Can you work these out from the model? Positions are in its coordinate system, mm. A direction names the side the tool comes from. Coordinates: 2 decimals unless noted, no trailing zeros. Loops run counter-clockwise (first coordinate to the right, second up) from the corner with the lowest first, then second, coordinate; pieces in that order, holes last. Notation, with made-up numbers: (59, 11) -> (86, 11) arc R32 cw to (86, 38) -> close; hole circle Ø7 at (-32, 2). An arc over 180 degrees is marked (long way). Use one line per item in the form item = value. Start each with the question number.
(1) I'm going to push flat-ended pins straight in: pin 1 (2 mm diameter, centred on y = -2, z = -18.5, fed in from +X); pin 2 (3 mm diameter, centred on y = 0, z = -3, fed in from +X); pin 3 (8 mm diameter, centred on y = -4.5, z = -2, fed in from -X); pin 4 (11.5 mm diameter, centred on x = 7, y = -1.5, fed in from -Z). Where does each tip first touch, or does it pass through?
(2) Imagine slicing it at C-C (x = -4). List the corners of the cut face in (y, z) for me.
(3) Imagine slicing it at A-A (z = -9). State how many separate pieces and enclosed holes the cut face has, plus the area to 3 significant figures.
(4) On a 3-axis mill with a long thin cutter (end or side, diameter ignored), from which of +Z, -Z, +X, -X, +Y, -Y can I reach the whole of each face in a straight line? I mean faces 1 (the flat face through (0, -9.5, -7)), 2 (the cylindrical face through (13.215, 9.199, -6.902)), 3 (the flat face through (5.5, -5, -22)), 4 (the flat face through (-6, -2, -7)). Say none if no direction works.
(5) Thinking about a two-plate mould opening in X: for faces 5 (the cylindrical face through (-14.45, -11.38, 1.52)), 6 (the flat face through (1.5, 5, -22)), 7 (the flat face through (1, 2, -6)), which applies, released by +X, released by -X, zero draft, split by the parting line, or undercut?
(6) I need wall thicknesses on line 1 (X direction, y = -7.5, z = -6); line 2 (Z direction, x = 18.5, y = 3.5); line 3 (X direction, y = 0.5, z = -15). Which ranges of each line are inside material? Lowest first, please. Write a range as [from, to].
(7) Imagine slicing it at B-B (z = -20). List the corners of the cut face in (x, y) for me.
(8) Imagine slicing it at D-D (x = 20). List the corners of the cut face in (y, z) for me, plus the area to 3 significant figures.
```python
from build123d import *
from OCP.BRepFilletAPI import BRepFilletAPI_MakeChamfer

# Parameters (mm, degrees)
SKIZZE1_R                       = 1.5
AUFSATZ_LINEAR_AUSTRAGEN1_DEPTH = 3
VERRUNDUNG1_R                   = 2
FASE1_SIZE                      = 1.5
AUFSATZ_LINEAR_AUSTRAGEN2_DEPTH = 2
AUFSATZ_LINEAR_AUSTRAGEN3_DEPTH = 14
SCHNITT_LINEAR_AUSTRAGEN1_DEPTH = 17
SKIZZE5_W                       = 24
SKIZZE5_H                       = 11
AUFSATZ_LINEAR_AUSTRAGEN4_DEPTH = 4
SKIZZE6_W                       = 3
SKIZZE6_H                       = 1
AUFSATZ_LINEAR_AUSTRAGEN5_DEPTH = 8
SKIZZE7_W                       = 2
SKIZZE7_H                       = 4
AUFSATZ_LINEAR_AUSTRAGEN6_DEPTH = 13
SKIZZE8_W                       = 2
SKIZZE8_H                       = 4
AUFSATZ_LINEAR_AUSTRAGEN7_DEPTH = 15
FASE2_SIZE                      = 2
FASE2_SIZE2                     = 0.75
VERRUNDUNG2_R                   = 0.25


with BuildPart() as part:
    # Skizze1 → Aufsatz-Linear austragen1 (new body)
    with BuildSketch(Plane.XY):
        with BuildLine():
            ThreePointArc((23.364069952, 3.949125596), (25.187731645, 0), (23.364069952, -3.949125596))
            Line((23.364069952, -3.949125596), (14.5, -11.5))
            Line((14.5, -11.5), (-14.5, -11.5))
            Line((-14.5, -11.5), (-23.364069952, -3.949125596))
            ThreePointArc((-23.364069952, -3.949125596), (-25.187731645, 0), (-23.364069952, 3.949125596))
            Line((-23.364069952, 3.949125596), (-14.5, 11.5))
            Line((-14.5, 11.5), (14.5, 11.5))
            Line((14.5, 11.5), (23.364069952, 3.949125596))
        make_face()
        with Locations((20, 0)):
            Circle(SKIZZE1_R, mode=Mode.SUBTRACT)
        with Locations((-20, 0)):
            Circle(SKIZZE1_R, mode=Mode.SUBTRACT)
    extrude(amount=AUFSATZ_LINEAR_AUSTRAGEN1_DEPTH)

    # Verrundung1
    verrundung1_edges = [part.edges().sort_by_distance(p)[0] for p in [
        (14.5, -11.5, 1.5),
        (-14.5, -11.5, 1.5),
        (-14.5, 11.5, 1.5),
        (14.5, 11.5, 1.5),
    ]]
    fillet(verrundung1_edges, radius=VERRUNDUNG1_R)

    # Fase1
    fase1_edges = [part.edges().sort_by_distance(p)[0] for p in [
        (18.5, 0, 3),
        (-21.5, 0, 3),
    ]]
    chamfer(fase1_edges, length=FASE1_SIZE)

    # Skizze2 → Aufsatz-Linear austragen2 (add)
    with BuildSketch(Plane.XY.offset(3)):
        with BuildLine():
            Line((-12.5, -11.5), (12.5, -11.5))
            ThreePointArc((12.5, -11.5), (14.621320344, -10.621320344), (15.5, -8.5))
            Line((15.5, -8.5), (15.5, 8.5))
            ThreePointArc((15.5, 8.5), (14.621320344, 10.621320344), (12.5, 11.5))
            Line((12.5, 11.5), (-12.5, 11.5))
            ThreePointArc((-12.5, 11.5), (-14.621320344, 10.621320344), (-15.5, 8.5))
            Line((-15.5, 8.5), (-15.5, -8.5))
            ThreePointArc((-15.5, -8.5), (-14.621320344, -10.621320344), (-12.5, -11.5))
        make_face()
    extrude(amount=AUFSATZ_LINEAR_AUSTRAGEN2_DEPTH)

    # Skizze4 → Aufsatz-Linear austragen3 (add)
    with BuildSketch(Plane(origin=(0, 0, 0), x_dir=(-1, 0, 0), z_dir=(0, 0, -1))):
        with BuildLine():
            Line((12.5, -9.5), (-12.5, -9.5))
            ThreePointArc((-12.5, -9.5), (-13.207106781, -9.207106781), (-13.5, -8.5))
            Line((-13.5, -8.5), (-13.5, 8.5))
            ThreePointArc((-13.5, 8.5), (-13.207106781, 9.207106781), (-12.5, 9.5))
            Line((-12.5, 9.5), (12.5, 9.5))
            ThreePointArc((12.5, 9.5), (13.207106781, 9.207106781), (13.5, 8.5))
            Line((13.5, 8.5), (13.5, -8.5))
            ThreePointArc((13.5, -8.5), (13.207106781, -9.207106781), (12.5, -9.5))
        make_face()
    extrude(amount=AUFSATZ_LINEAR_AUSTRAGEN3_DEPTH)

    # Skizze3 → Schnitt-Linear austragen1 (cut)
    with BuildSketch(Plane.XY.offset(5)):
        with BuildLine():
            Line((11.5, -8), (-11.5, -8))
            ThreePointArc((-11.5, -8), (-11.853553391, -7.853553391), (-12, -7.5))
            Line((-12, -7.5), (-12, 2.792893219))
            ThreePointArc((-12, 2.792893219), (-11.961939766, 2.984234935), (-11.853553391, 3.146446609))
            Line((-11.853553391, 3.146446609), (-7.146446609, 7.853553391))
            ThreePointArc((-7.146446609, 7.853553391), (-6.984234935, 7.961939766), (-6.792893219, 8))
            Line((-6.792893219, 8), (6.792893219, 8))
            ThreePointArc((6.792893219, 8), (6.984234935, 7.961939766), (7.146446609, 7.853553391))
            Line((7.146446609, 7.853553391), (11.853553391, 3.146446609))
            ThreePointArc((11.853553391, 3.146446609), (11.961939766, 2.984234935), (12, 2.792893219))
            Line((12, 2.792893219), (12, -7.5))
            ThreePointArc((12, -7.5), (11.853553391, -7.853553391), (11.5, -8))
        make_face()
    extrude(amount=-SCHNITT_LINEAR_AUSTRAGEN1_DEPTH, mode=Mode.SUBTRACT)

    # Skizze5 → Aufsatz-Linear austragen4 (add)
    with BuildSketch(Plane(origin=(0, 0, -14), x_dir=(-1, 0, 0), z_dir=(0, 0, -1))):
        Rectangle(SKIZZE5_W, SKIZZE5_H)
    extrude(amount=AUFSATZ_LINEAR_AUSTRAGEN4_DEPTH)

    # Skizze6 → Aufsatz-Linear austragen5 (add)
    with BuildSketch(Plane(origin=(0, 0, -18), x_dir=(-1, 0, 0), z_dir=(0, 0, -1))):
        with Locations((0, 5)):
            Rectangle(SKIZZE6_W, SKIZZE6_H)
        with Locations((-7, -5)):
            Rectangle(SKIZZE6_W, SKIZZE6_H)
        with Locations((7, -5)):
            Rectangle(SKIZZE6_W, SKIZZE6_H)
    extrude(amount=AUFSATZ_LINEAR_AUSTRAGEN5_DEPTH)

    # Skizze7 → Aufsatz-Linear austragen6 (add)
    with BuildSketch(Plane.XY.offset(-12)):
        with Locations((-7, -2)):
            Rectangle(SKIZZE7_W, SKIZZE7_H)
        with Locations((7, -2)):
            Rectangle(SKIZZE7_W, SKIZZE7_H)
    extrude(amount=AUFSATZ_LINEAR_AUSTRAGEN6_DEPTH)

    # Skizze8 → Aufsatz-Linear austragen7 (add)
    with BuildSketch(Plane.XY.offset(-12)):
        with Locations((0, 2)):
            Rectangle(SKIZZE8_W, SKIZZE8_H)
    extrude(amount=AUFSATZ_LINEAR_AUSTRAGEN7_DEPTH)

    # Fase2: one chamfer whose edges measure the first distance from different faces: ONE call of the kernel's chamfer builder (chamfer() names one face for all edges)
    fase2_edges_1 = [part.edges().sort_by_distance(p)[0] for p in [
        (7, -4, 1),
    ]]
    fase2_side_1 = [part.faces().sort_by_distance(p)[0] for p in [
        (7, -4, -5.5),
    ]]
    fase2_edges_2 = [part.edges().sort_by_distance(p)[0] for p in [
        (6, -2, 1),
    ]]
    fase2_side_2 = [part.faces().sort_by_distance(p)[0] for p in [
        (6, -2, -5.5),
    ]]
    fase2_edges_3 = [part.edges().sort_by_distance(p)[0] for p in [
        (7, 0, 1),
    ]]
    fase2_side_3 = [part.faces().sort_by_distance(p)[0] for p in [
        (7, 0, -5.5),
    ]]
    fase2_edges_4 = [part.edges().sort_by_distance(p)[0] for p in [
        (8, -2, 1),
    ]]
    fase2_side_4 = [part.faces().sort_by_distance(p)[0] for p in [
        (8, -2, -5.5),
    ]]
    fase2_edges_5 = [part.edges().sort_by_distance(p)[0] for p in [
        (0, 0, 3),
    ]]
    fase2_side_5 = [part.faces().sort_by_distance(p)[0] for p in [
        (0, 0, -4.5),
    ]]
    fase2_edges_6 = [part.edges().sort_by_distance(p)[0] for p in [
        (-1, 2, 3),
    ]]
    fase2_side_6 = [part.faces().sort_by_distance(p)[0] for p in [
        (-1, 2, -4.5),
    ]]
    fase2_edges_7 = [part.edges().sort_by_distance(p)[0] for p in [
        (0, 4, 3),
    ]]
    fase2_side_7 = [part.faces().sort_by_distance(p)[0] for p in [
        (0, 4, -4.5),
    ]]
    fase2_edges_8 = [part.edges().sort_by_distance(p)[0] for p in [
        (1, 2, 3),
    ]]
    fase2_side_8 = [part.faces().sort_by_distance(p)[0] for p in [
        (1, 2, -4.5),
    ]]
    fase2_edges_9 = [part.edges().sort_by_distance(p)[0] for p in [
        (-7, 0, 1),
    ]]
    fase2_side_9 = [part.faces().sort_by_distance(p)[0] for p in [
        (-7, 0, -5.5),
    ]]
    fase2_edges_10 = [part.edges().sort_by_distance(p)[0] for p in [
        (-6, -2, 1),
    ]]
    fase2_side_10 = [part.faces().sort_by_distance(p)[0] for p in [
        (-6, -2, -5.5),
    ]]
    fase2_edges_11 = [part.edges().sort_by_distance(p)[0] for p in [
        (-7, -4, 1),
    ]]
    fase2_side_11 = [part.faces().sort_by_distance(p)[0] for p in [
        (-7, -4, -5.5),
    ]]
    fase2_edges_12 = [part.edges().sort_by_distance(p)[0] for p in [
        (-8, -2, 1),
    ]]
    fase2_side_12 = [part.faces().sort_by_distance(p)[0] for p in [
        (-8, -2, -5.5),
    ]]
    fase2 = BRepFilletAPI_MakeChamfer(part.part.solid().wrapped)
    for e in fase2_edges_1:
        fase2.Add(FASE2_SIZE, FASE2_SIZE2, e.wrapped, fase2_side_1[0].wrapped)  # the first distance lies on this face
    for e in fase2_edges_2:
        fase2.Add(FASE2_SIZE, FASE2_SIZE2, e.wrapped, fase2_side_2[0].wrapped)  # the first distance lies on this face
    for e in fase2_edges_3:
        fase2.Add(FASE2_SIZE, FASE2_SIZE2, e.wrapped, fase2_side_3[0].wrapped)  # the first distance lies on this face
    for e in fase2_edges_4:
        fase2.Add(FASE2_SIZE, FASE2_SIZE2, e.wrapped, fase2_side_4[0].wrapped)  # the first distance lies on this face
    for e in fase2_edges_5:
        fase2.Add(FASE2_SIZE, FASE2_SIZE2, e.wrapped, fase2_side_5[0].wrapped)  # the first distance lies on this face
    for e in fase2_edges_6:
        fase2.Add(FASE2_SIZE, FASE2_SIZE2, e.wrapped, fase2_side_6[0].wrapped)  # the first distance lies on this face
    for e in fase2_edges_7:
        fase2.Add(FASE2_SIZE, FASE2_SIZE2, e.wrapped, fase2_side_7[0].wrapped)  # the first distance lies on this face
    for e in fase2_edges_8:
        fase2.Add(FASE2_SIZE, FASE2_SIZE2, e.wrapped, fase2_side_8[0].wrapped)  # the first distance lies on this face
    for e in fase2_edges_9:
        fase2.Add(FASE2_SIZE, FASE2_SIZE2, e.wrapped, fase2_side_9[0].wrapped)  # the first distance lies on this face
    for e in fase2_edges_10:
        fase2.Add(FASE2_SIZE, FASE2_SIZE2, e.wrapped, fase2_side_10[0].wrapped)  # the first distance lies on this face
    for e in fase2_edges_11:
        fase2.Add(FASE2_SIZE, FASE2_SIZE2, e.wrapped, fase2_side_11[0].wrapped)  # the first distance lies on this face
    for e in fase2_edges_12:
        fase2.Add(FASE2_SIZE, FASE2_SIZE2, e.wrapped, fase2_side_12[0].wrapped)  # the first distance lies on this face
    add(Compound.cast(fase2.Shape()), mode=Mode.REPLACE)

    # Verrundung2
    verrundung2_edges = [part.edges().sort_by_distance(p)[0] for p in [
        (1.5, 5, -26),
        (0, 4.5, -26),
        (-1.5, 5, -26),
        (0, 5.5, -26),
        (5.5, -5, -26),
        (7, -4.5, -26),
        (8.5, -5, -26),
        (7, -5.5, -26),
        (-5.5, -5, -26),
        (-7, -5.5, -26),
        (-8.5, -5, -26),
        (-7, -4.5, -26),
    ]]
    fillet(verrundung2_edges, radius=VERRUNDUNG2_R)


solid = part.part
```
Worked out:
q1.pin_1 = 12
q1.pin_2 = 13.5
q1.pin_3 = -25.08
q1.pin_4 = -26
q2.outline = (-11.5, 0) -> (-9.5, 0) -> (-9.5, -14) -> (-5.5, -14) -> (-5.5, -18) -> (5.5, -18) -> (5.5, -14) -> (9.5, -14) -> (9.5, 0) -> (11.5, 0) -> (11.5, 5) -> (8, 5) -> (8, -12) -> (-8, -12) -> (-8, 5) -> (-11.5, 5) -> close
q3.separate_pieces = 4
q3.enclosed_holes = 1
q3.area = 177 mm2
q4.face_1 = -Z, +X, -X, -Y
q4.face_2 = -Z, +X, +Y
q4.face_3 = -Z, +Y, -Y
q4.face_4 = +Z
q5.face_5 = released by -X
q5.face_6 = released by +X
q5.face_7 = undercut
q6.line_1 = [-13.5, -12], [12, 13.5]
q6.line_2 = [0, 3]
q6.line_3 = [-12, 12]
q7.outline = (-8.5, -5.5) -> (-5.5, -5.5) -> (-5.5, -4.5) -> (-8.5, -4.5) -> close; (-1.5, 4.5) -> (1.5, 4.5) -> (1.5, 5.5) -> (-1.5, 5.5) -> close; (5.5, -5.5) -> (8.5, -5.5) -> (8.5, -4.5) -> (5.5, -4.5) -> close
q8.outline = (-6.81, 0) -> (-1.5, 0) -> (-1.5, 1.5) -> (-3, 3) -> (-6.81, 3) -> close; (1.5, 0) -> (6.81, 0) -> (6.81, 3) -> (3, 3) -> (1.5, 1.5) -> close
q8.area = 29.6 mm2
